Verification items for this drawing (mm, ordinates from the low corner). Give positions to 0.01 mm unless a question says otherwise; leave off trailing zeros. Loops run counter-clockwise (first coordinate to the right, second up) from the corner with the lowest first, then second, coordinate; pieces in that order, holes last. Notation, with made-up numbers: (-37.75, 73) -> (-5.75, 73) arc R21 cw to (-5.75, 109) -> close; hole circle Ø11 at (10, 78). An arc over 180 degrees is marked (long way). Write item = value, one per line.
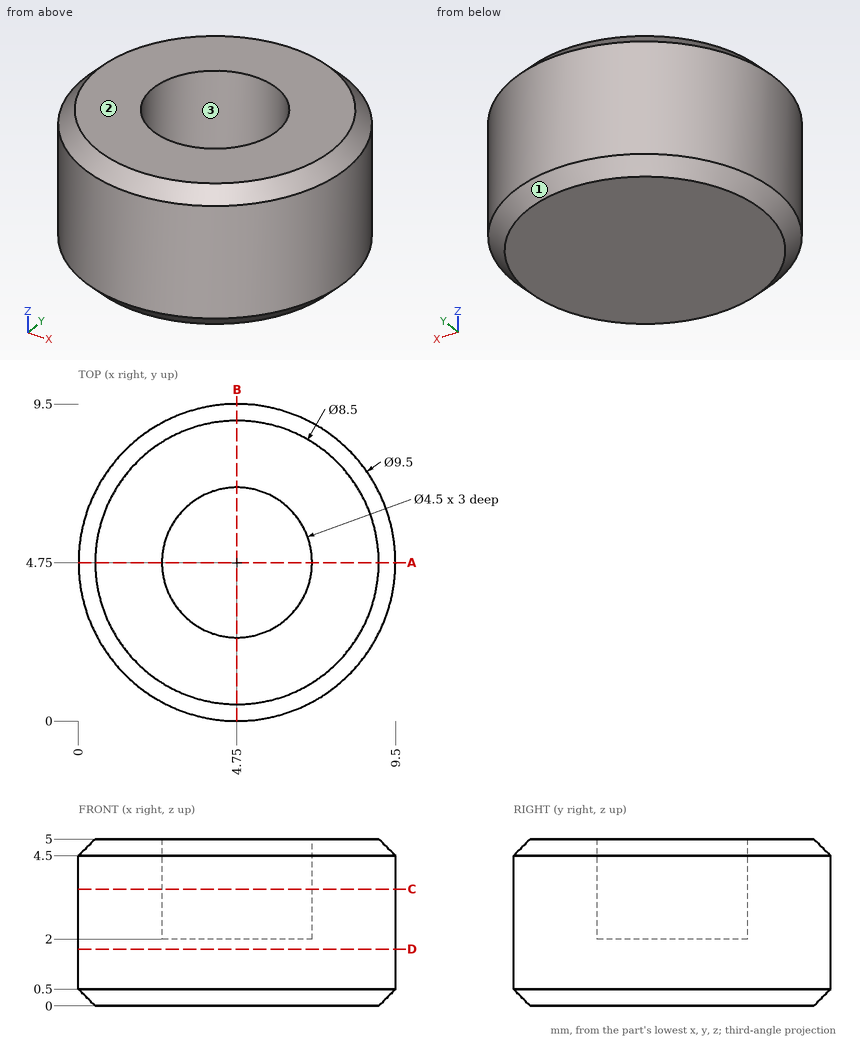
Item 1: Section check A-A, the plane y = 4.75. Record the cut outline in (x, z), plus the area to 3 significant figures.
Answer:
outline = (0, 0.5) -> (0.5, 0) -> (9, 0) -> (9.5, 0.5) -> (9.5, 4.5) -> (9, 5) -> (7, 5) -> (7, 2) -> (2.5, 2) -> (2.5, 5) -> (0.5, 5) -> (0, 4.5) -> close
area = 33.5 mm^2
Item 2: Draft check along Y on the marked faces 1, 2 and 3. Enter one of: +Y half, -Y half, draft (parallel to the pull), parting line (faces both ways), or undercut.
Answer:
face_1 = parting line
face_2 = draft
face_3 = undercut
Item 3: Section check D-D, the plane z = 1.7. Record the cut outline in (x, y), plus the area to 3 significant figures.
Answer:
outline = circle Ø9.5 at (4.75, 4.75)
area = 70.9 mm^2
Item 4: Thickness scan on L1, parallel to Y at x = 4.75, z = 3.65; L2, parallel to X at y = 6.5, z = 2.25; L3, parallel to X at y = 4.5, z = 4.3. Record the ranges inside material, lowest first. Write a range as [from, to].
Answer:
L1 = [0, 2.5], [7, 9.5]
L2 = [0.33, 3.34], [6.16, 9.17]
L3 = [0.01, 2.51], [6.99, 9.49]
Item 5: Gauge pin test, flat end, axial feed: pin 1 (3.5 mm diameter, centred on x = 4.5, y = 4.5, fed in from +Z). Record the tip position at first contact, or that the pin passes through.
Answer:
pin_1 = 2
Item 6: Section check C-C, the plane z = 3.5. Record the cut outline in (x, y).
Answer:
outline = circle Ø9.5 at (4.75, 4.75); hole circle Ø4.5 at (4.75, 4.75)
